Source: CAD feature listing. Evaluate the final solid. Frame: model axes, mm. A direction names the side the tool comes from. Coordinates: 2 decimals unless noted, no trailing zeros. Write each loop counter-clockwise with the first axis right and the second up, starting at its lowest first coordinate (ties: lowest second). Pieces come first, ordered by that corner, then holes. Notation, with made-up numbers: (-36.75, -26.75) -> (9.25, -26.75) arc R26 cw to (9.25, 4.25) -> close; hole circle Ø1 at (-37.5, -21.75). An arc over 180 degrees is marked (long way). One line per item, written item: value. Start each with the question number.
1. Section query B-B, the plane z = 2. Output: boundary loops of the cut face in (x, y), and give its area (3 significant figures).
2. First-contact query: P1, Ø6, axis at y = -12, z = 1.5, coming from the -X side; P2, Ø20, axis at x = 0, y = 0, coming from the +Z side; P3, Ø12, axis at y = -0.5, z = 1.5, coming from the +X side; P4, Ø4, axis at y = -7.5, z = 2, coming from the -X side. Flat tips, straight axial feed; report the tip coordinate or a pass-through.
3. Section query A-A, the plane y = 15. Output: boundary loops of the cut face in (x, z).
4. Line query: line 1 (X direction, y = 0, z = -10.2); line 2 (Y direction, x = 0, z = -10.35); line 3 (Z direction, x = 3.5, y = 9.5). Output: solid intervals per line, ascending.
5. Section query D-D, the plane y = -10. Output: boundary loops of the cut face in (x, z), and give its area (3 significant figures).
6. Mould query, pull axis Z, two halves, no side actions, for faces 1 (the cylindrical face through (-0.227, -6.246, -3.819)), 2 (the cylindrical face through (-3, -0.1, -10.2)), 3 (the flat face through (0, -4, 4)). Classes: released by +Z, released by -Z, zero draft, split by the parting line, or undercut.
7. Access query for faces 4 (the cylindrical face through (10.877, -11.686, 5.479)), 5 (the flat face through (0, 4, -10)), 6 (the cylindrical face through (2.58, -4.05, -17.26)). Directions: +Z, -Z, +X, -X, +Y, -Y. A direction counts if a zero-diameter tool reaches every point of the face in a straight line with its end or side. Return the directions, or none.
8. Section query C-C, the plane x = 10. Output: boundary loops of the cut face in (y, z), and give its area (3 significant figures).
from build123d import *

# Parameters (mm, degrees)
F0_R      = 1.9
F1_DEPTH  = 4
F2_DEPTH  = 7
F4_DEPTH  = 5
F6_DEPTH  = 5
F7_R      = 3
F8_DEPTH  = 8
F9_R      = 4.8
F9_R_2    = 4.1
F10_DEPTH = 1.5
F9_R_3    = 3
F11_DEPTH = 7.5


with BuildPart() as f1:
    # F0 (on Top) → F1 (new body)
    with BuildSketch(Plane.XY):
        with BuildLine():
            ThreePointArc((-3.25, 19.7341708719), (-12.9421791055, -15.247950682), (20, 0))
            ThreePointArc((20, 0), (15.247950682, 12.9421791055), (3.25, 19.7341708719))
            Line((3.25, 19.7341708719), (3.25, 0))
            ThreePointArc((3.25, 0), (0, -3.25), (-3.25, 0))
            Line((-3.25, 0), (-3.25, 19.7341708719))
        make_face()
        with Locations((-10, -10)):
            Circle(F0_R, mode=Mode.SUBTRACT)
        with Locations((10, -10)):
            Circle(F0_R, mode=Mode.SUBTRACT)
        with Locations((-10, 10)):
            Circle(F0_R, mode=Mode.SUBTRACT)
        with Locations((10, 10)):
            Circle(F0_R, mode=Mode.SUBTRACT)
        with Locations((-10, 10)):
            Circle(F0_R)
        with Locations((10, 10)):
            Circle(F0_R)
        with Locations((10, -10)):
            Circle(F0_R)
        with Locations((-10, -10)):
            Circle(F0_R)
    extrude(amount=F1_DEPTH)

    # F0 (on Top) → F2 (join)
    with BuildSketch(Plane.XY):
        with Locations((-10, 10)):
            Circle(F0_R)
        with Locations((10, 10)):
            Circle(F0_R)
        with Locations((10, -10)):
            Circle(F0_R)
        with Locations((-10, -10)):
            Circle(F0_R)
    extrude(amount=F2_DEPTH)

    # F3 (on face) → F4 (join)
    with BuildSketch(Plane(origin=(0, 0, 0), x_dir=(1, 0, 0), z_dir=(0, 0, -1))):
        with BuildLine():
            ThreePointArc((-3.25, -5.338539126), (-3.0618621785, 5.4486236794), (6.25, 0))
            ThreePointArc((6.25, 0), (5.4486236794, -3.0618621785), (3.25, -5.338539126))
            Line((3.25, -5.338539126), (3.25, -12.3031496292))
            Line((3.25, -12.3031496292), (12.2798401255, -7.0897690021))
            Line((12.2798401255, -7.0897690021), (12.2798401255, 7.0897690021))
            Line((12.2798401255, 7.0897690021), (0, 14.1795380041))
            Line((0, 14.1795380041), (-12.2798401255, 7.0897690021))
            Line((-12.2798401255, 7.0897690021), (-12.2798401255, -7.0897690021))
            Line((-12.2798401255, -7.0897690021), (-3.25, -12.3031496292))
            Line((-3.25, -12.3031496292), (-3.25, -5.338539126))
        make_face()
    extrude(amount=F4_DEPTH)

    # F5 (on face) → F6 (join)
    with BuildSketch(Plane(origin=(0, 0, -5), x_dir=(1, 0, 0), z_dir=(0, 0, -1))):
        with BuildLine():
            ThreePointArc((-6.25, 0), (0, 6.25), (6.25, 0))
            Line((6.25, 0), (6.25, -10.5710988217))
            Line((6.25, -10.5710988217), (12.2798401255, -7.0897690021))
            Line((12.2798401255, -7.0897690021), (12.2798401255, 7.0897690021))
            Line((12.2798401255, 7.0897690021), (0, 14.1795380041))
            Line((0, 14.1795380041), (-12.2798401255, 7.0897690021))
            Line((-12.2798401255, 7.0897690021), (-12.2798401255, -7.0897690021))
            Line((-12.2798401255, -7.0897690021), (-6.25, -10.5710988217))
            Line((-6.25, -10.5710988217), (-6.25, 0))
        make_face()
    extrude(amount=F6_DEPTH)

    # F7 (on face) → F8 (join)
    with BuildSketch(Plane(origin=(0, 0, -10), x_dir=(1, 0, 0), z_dir=(0, 0, -1))):
        with BuildLine():
            ThreePointArc((-6.2500000608, 0), (-7.83e-08, 6.2500000351), (6.2499999392, 3.51e-08))
            Line((6.25, 0), (6.25, -10.5710988217))
            Line((6.2499999696, -10.571098769), (12.2798400647, -7.089768967))
            Line((12.2798400647, -7.089768967), (12.2798400647, 7.0897690371))
            Line((12.2798400647, 7.0897690371), (-6.08e-08, 14.1795380392))
            Line((-6.08e-08, 14.1795380392), (-12.2798401862, 7.0897690371))
            Line((-12.2798401862, 7.0897690371), (-12.2798401862, -7.089768967))
            Line((-12.2798401862, -7.089768967), (-6.25, -10.5710988217))
            Line((-6.25, -10.5710988217), (-6.25, 0))
        make_face()
        with BuildLine():
            ThreePointArc((-6.2500000608, 0), (-4.32e-08, -6.2499999649), (6.2499999392, 3.51e-08))
            ThreePointArc((6.2499999392, 3.51e-08), (-7.83e-08, 6.2500000351), (-6.2500000608, 0))
        make_face()
        with Locations((-6.08e-08, 3.51e-08)):
            Circle(F7_R, mode=Mode.SUBTRACT)
        with BuildLine():
            Line((6.25, -10.5710988217), (6.25, 0))
            ThreePointArc((6.2499999392, 3.51e-08), (-4.32e-08, -6.2499999649), (-6.2500000608, 0))
            Line((-6.25, 0), (-6.25, -10.5710988217))
            Line((-6.25, -10.5710988217), (-6.08e-08, -14.179537969))
            Line((-6.08e-08, -14.179537969), (6.2499999696, -10.571098769))
        make_face()
    extrude(amount=F8_DEPTH)

    # F9 (on face) → F10 (cut)
    with BuildSketch(Plane(origin=(0, 0, -18), x_dir=(1, 0, 0), z_dir=(0, 0, -1))):
        with Locations((-6.08e-08, 3.51e-08)):
            Circle(F9_R)
        with Locations((-6.08e-08, 3.51e-08)):
            Circle(F9_R_2, mode=Mode.SUBTRACT)
    extrude(amount=-F10_DEPTH, mode=Mode.SUBTRACT)

    # F9 (on face) → F11 (cut)
    with BuildSketch(Plane(origin=(0, 0, -18), x_dir=(1, 0, 0), z_dir=(0, 0, -1))):
        with Locations((-6.08e-08, 3.51e-08)):
            Circle(F9_R_2)
        with Locations((-6.08e-08, 3.51e-08)):
            Circle(F9_R_3, mode=Mode.SUBTRACT)
    extrude(amount=-F11_DEPTH, mode=Mode.SUBTRACT)


solid = f1.part
Computed values:
1. outline: (-3.25, 0) -> (-3.25, 19.73) arc R20 ccw (long way) to (3.25, 19.73) -> (3.25, 0) arc R3.25 cw to start
1. area: 1,110 mm²
2. P1: stops at x = -17.86
2. P2: stops at z = 4
2. P3: stops at x = 20
2. P4: stops at x = -19.23
3. outline: (-13.23, 0) -> (-3.25, 0) -> (-3.25, 4) -> (-13.23, 4) -> close; (3.25, 0) -> (13.23, 0) -> (13.23, 4) -> (3.25, 4) -> close
4. line 1: x = -12.28 to -3, 3 to 12.28
4. line 2: y = -14.18 to -3, 3 to 14.18
4. line 3: z = -18 to -10, -5 to 4
5. outline: (-17.32, 0) -> (-7.24, 0) -> (-7.24, -18) -> (7.24, -18) -> (7.24, 0) -> (17.32, 0) -> (17.32, 4) -> (11.9, 4) -> (11.9, 7) -> (8.1, 7) -> (8.1, 4) -> (-8.1, 4) -> (-8.1, 7) -> (-11.9, 7) -> (-11.9, 4) -> (-17.32, 4) -> close
5. area: 422 mm²
6. face 1: undercut
6. face 2: zero draft
6. face 3: released by +Z
7. face 4: +Z
7. face 5: +Y
7. face 6: -Z
8. outline: (-17.32, 0) -> (-8.41, 0) -> (-8.41, -18) -> (8.41, -18) -> (8.41, 0) -> (17.32, 0) -> (17.32, 4) -> (11.9, 4) -> (11.9, 7) -> (8.1, 7) -> (8.1, 4) -> (-8.1, 4) -> (-8.1, 7) -> (-11.9, 7) -> (-11.9, 4) -> (-17.32, 4) -> close
8. area: 464 mm²
